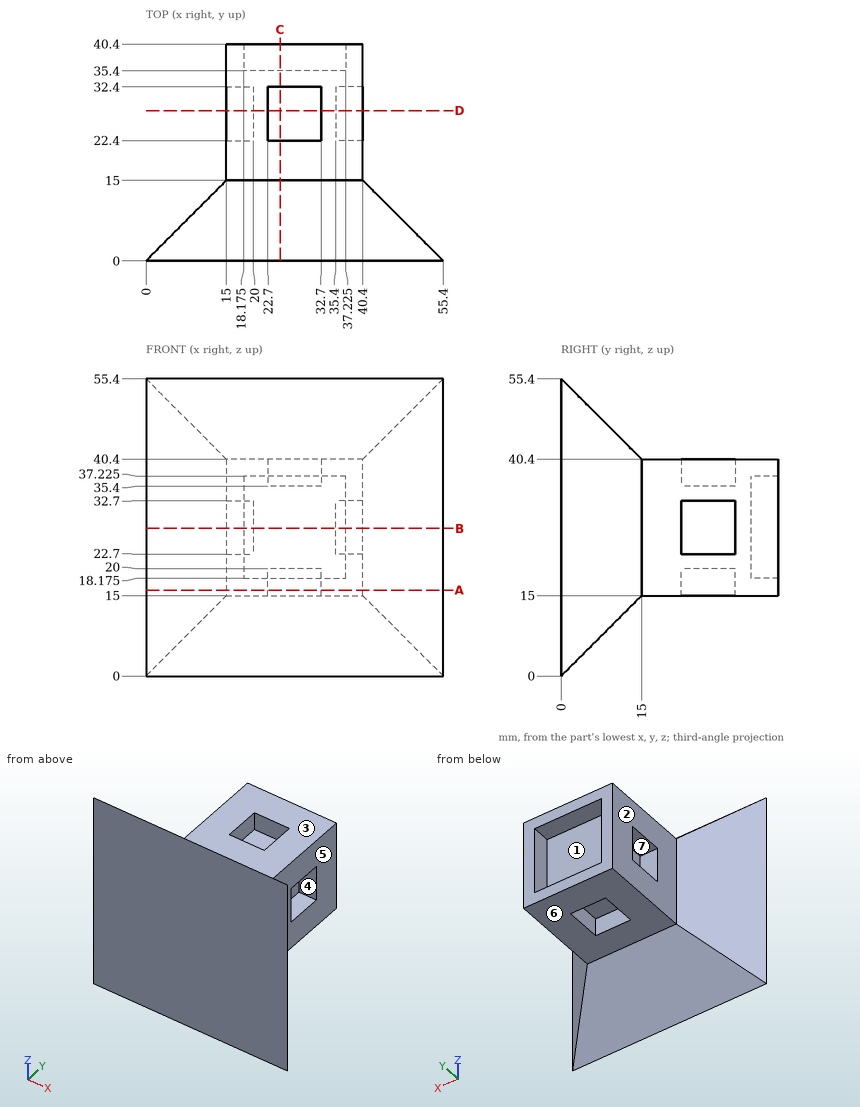
Drawing for the job (mm, zero at the part's lowest x, y, z). A direction names the side the tool comes from. Round coordinates to 2 decimals unless told otherwise and drop trailing zeros. Write each loop counter-clockwise with the first axis right and the second up, starting at its lowest first coordinate (ties: lowest second). Pieces come first, ordered by that corner, then holes. Notation, with made-up numbers: M 58.25,-23.5 L 91.25,-23.5 A5 cw 91.25,-14.5 Z; hole C 62,37.5 d6. An arc over 180 degrees is marked long. Answer in a Markdown table with one row per item.
1. Saw through at B-B (z = 27.5). List the corners of the cut face in (x, y) (3 decimals).
Geometry check:
| item | result |
|---|---|
| outline | M 0,0 L 55.4,0 L 40.4,15 L 40.4,22.4 L 35.4,22.4 L 35.4,32.4 L 40.4,32.4 L 40.4,40.4 L 37.225,40.4 L 37.225,35.4 L 18.175,35.4 L 18.175,40.4 L 15,40.4 L 15,32.4 L 20,32.4 L 20,22.4 L 15,22.4 L 15,15 Z |
2. Which spindle directions (+Z, -Z, +X, -X, +Y, -Y) get a long thin tool onto all of the face, cutting with end or side? Do the marked faces 4, 5, 6 and 7. Say none if no direction does.
Geometry check:
| item | result |
|---|---|
| face 4 | +X |
| face 5 | +Z, -Z, +X, +Y |
| face 6 | -Z, +X, -X, +Y |
| face 7 | -X |
3. Flat gauge pins, fed straight in: P1, Ø12, axis at x = 17, y = 10, coming from the -Z side; P2, Ø11, axis at y = 29.5, z = 26, coming from the +X side; P3, Ø10, axis at x = 49, z = 42.5, coming from the +Y side. Where does each tip first touch, or does it go through?
Geometry check:
| item | result |
|---|---|
| P1 | z = 4 |
| P2 | x = 40.4 |
| P3 | y = 11.4 |
4. Saw through at D-D (y = 28). List the corners of the cut face in (x, z).
Geometry check:
| item | result |
|---|---|
| outline | M 15,15 L 22.7,15 L 22.7,20 L 32.7,20 L 32.7,15 L 40.4,15 L 40.4,22.7 L 35.4,22.7 L 35.4,32.7 L 40.4,32.7 L 40.4,40.4 L 32.7,40.4 L 32.7,35.4 L 22.7,35.4 L 22.7,40.4 L 15,40.4 L 15,32.7 L 20,32.7 L 20,22.7 L 15,22.7 Z |
5. Probe L1, parallel to X at y = 25, z = 18.5; L2, parallel to Z at x = 26, y = 37 (3 decimals); L3, parallel to X at y = 33.5, z = 36. List the from-to ranges inside material, lowest first. Write a range as [from, to].
Geometry check:
| item | result |
|---|---|
| L1 | [15, 22.7], [32.7, 40.4] |
| L2 | [15, 18.175], [37.225, 40.4] |
| L3 | [15, 40.4] |
6. Mould opens along Z. For the marked faces 1, 2 and 3 say: +Z half, -Z half, draft (parallel to the pull), parting line (faces both ways), or undercut.
Geometry check:
| item | result |
|---|---|
| face 1 | undercut |
| face 2 | draft |
| face 3 | +Z half |
7. Saw through at C-C (x = 25). List the corners of the cut face in (y, z) (3 decimals), and give its area (3 significant figures).
Geometry check:
| item | result |
|---|---|
| outline | M 0,0 L 15,15 L 22.4,15 L 22.4,20 L 32.4,20 L 32.4,15 L 40.4,15 L 40.4,18.175 L 35.4,18.175 L 35.4,37.225 L 40.4,37.225 L 40.4,40.4 L 32.4,40.4 L 32.4,35.4 L 22.4,35.4 L 22.4,40.4 L 15,40.4 L 0,55.4 Z |
| area | 1,060 mm2 |
8. Saw through at A-A (z = 16). List the corners of the cut face in (x, y), and give its area (3 significant figures).
Geometry check:
| item | result |
|---|---|
| outline | M 0,0 L 55.4,0 L 40.4,15 L 40.4,40.4 L 15,40.4 L 15,15 Z; hole M 22.7,22.4 L 32.7,22.4 L 32.7,32.4 L 22.7,32.4 Z |
| area | 1,150 mm2 |
